Work out the finished part from the listing and answer in its coordinate system (mm). A direction names the side the tool comes from. Give positions to 0.01 mm unless a question says otherwise; leave off trailing zeros. Order: outer loops, then holes, each group sorted by start corner. A loop starts at its lowest first (then second) coordinate and runs counter-clockwise, first axis right, second up. Notation, with made-up numbers: (53.25, 76) -> (81.25, 76) arc R37 ccw to (81.25, 113) -> close; hole circle Ø1 at (-24.75, -14.5). An arc over 180 degrees is marked (long way). Use a Markdown table: item, result. Add a question column.
```python
from build123d import *

# Parameters (mm, degrees)
SKETCH1_W           = 14.8
SKETCH1_H           = 8.08
BOSS_EXTRUDE1_DEPTH = 6.94
FILLET1_SIZE        = 7
FILLET1_SIZE_2      = 3.4
SKETCH2_W           = 2.5
SKETCH2_H           = 5
BOSS_EXTRUDE2_DEPTH = 7.45
SKETCH3_W           = 4.44
SKETCH3_H           = 5
BOSS_EXTRUDE3_DEPTH = 3
CUT_EXTRUDE1_REACH  = 26.161
CUT_EXTRUDE2_REACH  = 26.161
CUT_EXTRUDE3_REACH  = 25.756
SKETCH6_W           = 1.27
SKETCH6_H           = 10.45
SKETCH7_W           = 6.5278
SKETCH7_H           = 5
SKETCH7_H_2         = 1.3
BOSS_EXTRUDE4_DEPTH = 2.55634
CUT_EXTRUDE4_REACH  = 24.207
SKETCH9_W           = 6.5278
SKETCH9_H           = 8.018408457
SKETCH9_W_2         = 4.3283
SKETCH9_H_2         = 5.8777
BOSS_EXTRUDE5_DEPTH = 16.3863


with BuildPart() as part:
    # Sketch1 → Boss-Extrude1 (new body)
    with BuildSketch(Plane(origin=(0, 0, 0), x_dir=(1, 0, 0), z_dir=(0, 1, 0))):
        with BuildLine():
            Line((0, -8.08), (14.8, -8.08))
            ThreePointArc((14.8, -8.08), (7.4, -15.48), (0, -8.08))
        make_face()
        with Locations((7.4, -4.04)):
            Rectangle(SKETCH1_W, SKETCH1_H)
        with BuildLine():
            ThreePointArc((0, 0), (7.4, 7.4), (14.8, 0))
            Line((14.8, 0), (0, 0))
        make_face()
    extrude(amount=BOSS_EXTRUDE1_DEPTH)

    # Fillet1
    # an asymmetric fillet: 7, 3.4 mm, written as the material it takes off along each edge
    with BuildSketch(Plane(origin=(7.4, 6.94, 0), x_dir=(-1, 0, 0), z_dir=(0, 0, 1))) as fillet1_piece_1:
        with BuildLine():
            Bezier((7.4 - FILLET1_SIZE, 0), (7.4, 0), (7.4, FILLET1_SIZE_2), weights=[1, 0.707106781, 1])
            Line((7.4, FILLET1_SIZE_2), (7.4, 0))
            Line((7.4, 0), (7.4 - FILLET1_SIZE, 0))
        make_face()
    revolve(axis=Axis((7.4, 6.94, 0), (0, -1, 0)), revolution_arc=180, mode=Mode.SUBTRACT)
    with BuildSketch(Plane(origin=(0, 6.94, 8.08), x_dir=(0, -1, 0), z_dir=(0, 0, -1)), Plane(origin=(14.8, 6.94, 0), x_dir=(0, -1, 0), z_dir=(0, 0, 1))) as fillet1_piece_2:
        with BuildLine():
            Bezier((FILLET1_SIZE_2, 0), (0, 0), (0, -FILLET1_SIZE), weights=[1, 0.707106781, 1])
            Line((0, -FILLET1_SIZE), (0, 0))
            Line((0, 0), (FILLET1_SIZE_2, 0))
        make_face()
    extrude(amount=8.08, mode=Mode.SUBTRACT)
    with BuildSketch(Plane(origin=(7.4, 6.94, 8.08), x_dir=(1, 0, 0), z_dir=(0, 0, -1))) as fillet1_piece_3:
        with BuildLine():
            Bezier((7.4, FILLET1_SIZE_2), (7.4, 0), (7.4 - FILLET1_SIZE, 0), weights=[1, 0.707106781, 1])
            Line((7.4 - FILLET1_SIZE, 0), (7.4, 0))
            Line((7.4, 0), (7.4, FILLET1_SIZE_2))
        make_face()
    revolve(axis=Axis((7.4, 6.94, 8.08), (0, -1, 0)), revolution_arc=180, mode=Mode.SUBTRACT)

    # Sketch2 → Boss-Extrude2 (add)
    with BuildSketch(Plane.XZ):
        with Locations((1.25, 4.04)):
            Rectangle(SKETCH2_W, SKETCH2_H)
        with Locations((13.55, 4.04)):
            Rectangle(SKETCH2_W, SKETCH2_H)
    extrude(amount=BOSS_EXTRUDE2_DEPTH)

    # Sketch3 → Boss-Extrude3 (add)
    with BuildSketch(Plane(origin=(0, -7.45, 0), x_dir=(-1, 0, 0), z_dir=(0, -1, 0))):
        with Locations((-0.28, -4.04)):
            Rectangle(SKETCH3_W, SKETCH3_H)
        with Locations((-14.52, -4.04)):
            Rectangle(SKETCH3_W, SKETCH3_H)
    extrude(amount=BOSS_EXTRUDE3_DEPTH)

    # Sketch4 → Cut-Extrude1 (cut, up to next)
    with BuildSketch(Plane(origin=(0, 0, 1.54), x_dir=(-1, 0, 0), z_dir=(0, 0, -1)), mode=Mode.PRIVATE) as cut_extrude1_sk1:
        Polygon((1.94, -7.45), (-0.28, -10.45), (1.94, -10.45), align=None)
    cut_extrude1_tool1 = extrude(cut_extrude1_sk1.sketch, amount=-CUT_EXTRUDE1_REACH, mode=Mode.PRIVATE) & part.part
    # Sketch4 → Cut-Extrude1 (cut, up to next)
    with BuildSketch(Plane(origin=(0, 0, 1.54), x_dir=(-1, 0, 0), z_dir=(0, 0, -1)), mode=Mode.PRIVATE) as cut_extrude1_sk2:
        Polygon((-16.74, -7.45), (-16.74, -10.45), (-14.52, -10.45), align=None)
    cut_extrude1_tool2 = extrude(cut_extrude1_sk2.sketch, amount=-CUT_EXTRUDE1_REACH, mode=Mode.PRIVATE) & part.part
    add(cut_extrude1_tool1.solids().sort_by_distance((-1.2, -9.45, 1.54))[0], mode=Mode.SUBTRACT)
    add(cut_extrude1_tool2.solids().sort_by_distance((16, -9.45, 1.54))[0], mode=Mode.SUBTRACT)

    # Sketch5 → Cut-Extrude2 (cut, up to next)
    with BuildSketch(Plane(origin=(0, 0, 1.54), x_dir=(-1, 0, 0), z_dir=(0, 0, -1)), mode=Mode.PRIVATE) as cut_extrude2_sk1:
        Polygon((-0.28, -10.45), (-0.87, -10.45), (1.35, -7.45), (1.94, -7.45), align=None)
    cut_extrude2_tool1 = extrude(cut_extrude2_sk1.sketch, amount=-CUT_EXTRUDE2_REACH, mode=Mode.PRIVATE) & part.part
    # Sketch5 → Cut-Extrude2 (cut, up to next)
    with BuildSketch(Plane(origin=(0, 0, 1.54), x_dir=(-1, 0, 0), z_dir=(0, 0, -1)), mode=Mode.PRIVATE) as cut_extrude2_sk2:
        Polygon((-14.52, -10.45), (-13.93, -10.45), (-16.15, -7.45), (-16.74, -7.45), align=None)
    cut_extrude2_tool2 = extrude(cut_extrude2_sk2.sketch, amount=-CUT_EXTRUDE2_REACH, mode=Mode.PRIVATE) & part.part
    add(cut_extrude2_tool1.solids().sort_by_distance((-0.535, -8.95, 1.54))[0], mode=Mode.SUBTRACT)
    add(cut_extrude2_tool2.solids().sort_by_distance((15.335, -8.95, 1.54))[0], mode=Mode.SUBTRACT)

    # Sketch6 → Cut-Extrude3 (cut, up to next)
    with BuildSketch(Plane(origin=(0, 0, 1.54), x_dir=(-1, 0, 0), z_dir=(0, 0, -1)), mode=Mode.PRIVATE) as cut_extrude3_sk1:
        with Locations((-1.865, -5.225)):
            Rectangle(SKETCH6_W, SKETCH6_H)
    cut_extrude3_tool1 = extrude(cut_extrude3_sk1.sketch, amount=-CUT_EXTRUDE3_REACH, mode=Mode.PRIVATE) & part.part
    # Sketch6 → Cut-Extrude3 (cut, up to next)
    with BuildSketch(Plane(origin=(0, 0, 1.54), x_dir=(-1, 0, 0), z_dir=(0, 0, -1)), mode=Mode.PRIVATE) as cut_extrude3_sk2:
        with Locations((-12.935, -5.225)):
            Rectangle(SKETCH6_W, SKETCH6_H)
    cut_extrude3_tool2 = extrude(cut_extrude3_sk2.sketch, amount=-CUT_EXTRUDE3_REACH, mode=Mode.PRIVATE) & part.part
    add(cut_extrude3_tool1.solids().sort_by_distance((1.865, -5.225, 1.54))[0], mode=Mode.SUBTRACT)
    add(cut_extrude3_tool2.solids().sort_by_distance((12.935, -5.225, 1.54))[0], mode=Mode.SUBTRACT)

    # Sketch7 → Boss-Extrude4 (add)
    with BuildSketch(Plane.XZ):
        with Locations((7.3989, 4.04)):
            Rectangle(SKETCH7_W, SKETCH7_H)
        with Locations((7.3989, 0.89)):
            Rectangle(SKETCH7_W, SKETCH7_H_2)
        with Locations((7.3989, 7.19)):
            Rectangle(SKETCH7_W, SKETCH7_H_2)
    extrude(amount=BOSS_EXTRUDE4_DEPTH)

    # Sketch8 → Cut-Extrude4 (cut, up to next)
    with BuildSketch(Plane(origin=(10.6628, 0, 0), x_dir=(0, 0, -1), z_dir=(1, 0, 0)), mode=Mode.PRIVATE) as cut_extrude4_sk1:
        Polygon((-0.24, -2.55634), (-7.84, 0), (-7.84, -2.55634), align=None)
    cut_extrude4_tool1 = extrude(cut_extrude4_sk1.sketch, amount=-CUT_EXTRUDE4_REACH, mode=Mode.PRIVATE) & part.part
    add(cut_extrude4_tool1.solids().sort_by_distance((10.6628, -1.704227, 5.306667))[0], mode=Mode.SUBTRACT)

    # Sketch9 → Boss-Extrude5 (add)
    with BuildSketch(Plane(origin=(0, -2.369037415, 0.796850672), x_dir=(1, 0, 0), z_dir=(0, -0.9478190142131836, 0.31880890247285915))):
        with Locations((7.3989, 3.421696842)):
            Rectangle(SKETCH9_W, SKETCH9_H)
        with Locations((7.3989, 3.421696843)):
            Rectangle(SKETCH9_W_2, SKETCH9_H_2, mode=Mode.SUBTRACT)
    extrude(amount=BOSS_EXTRUDE5_DEPTH)


solid = part.part
```
1) The part is cut by section C-C, the plane y = 2. Determine the outline of the cut face in (x, z).
2) Flat-ended cylindrical pins translate along their axes: pin 1 (2 mm diameter, centred on x = 12, y = 1, fed in from +Z); pin 2 (4 mm diameter, centred on y = -6, z = 3, fed in from -X); pin 3 (4 mm diameter, centred on y = -10, z = 7.5, fed in from -X); pin 4 (1 mm diameter, centred on x = 3.5, y = -11, fed in from +Z). Find the tip coordinate at first contact, or state that the pin passes through.
3) The part is cut by section A-A, the plane y = -5.5. Determine the outline of the cut face in (x, z) (3 decimals).
4) Which of the six approach directions +Z, -Z, +X, -X, +Y, -Y give full straight-line access (tool end or side, diameter ignored) to faces 4 (the flat face through (5.235, -9, 7)), 5 (the flat face through (1.23, -5, 4)), 6 (the flat face through (7.353, -7.657, 10.415)), 7 (the flat face through (15, -7.45, 4))?
5) Straight lines are drawn through the part: line 1 (X direction, y = -3.75, z = 4.25) (3 decimals); line 2 (X direction, y = -9.75, z = 4.25) (3 decimals); line 3 (X direction, y = -9.5, z = 8.25) (3 decimals). For each, find the intervals that lie inside material, in ascending order.
6) The part is cut by section B-B, the plane y = -14.75. Determine the outline of the cut face in (x, z) (3 decimals), then the cut area to 3 significant figures.
7) Determine the mould class of faces 1 (the cylindrical face through (7.56, 1.75, 15.48)), 2 (the flat face through (9.563, -9, 7)), 3 (the flat face through (10.663, -8, 6)) for opening direction Z: released by +Z, released by -Z, zero draft, split by the parting line, or undercut.
A:
| question | item | result |
|---|---|---|
| 1 | outline | (0, 0) arc R7.4 ccw to (14.8, 0) -> (14.8, 8.08) arc R7.4 ccw to (0, 8.08) -> close |
| 2 | pin 1 | z = 14.55 |
| 2 | pin 2 | x = -1.35 |
| 2 | pin 3 | x = -0.76 |
| 2 | pin 4 | through |
| 3 | outline | (0, 1.54) -> (1.23, 1.54) -> (1.23, 6.54) -> (0, 6.54) -> close; (4.135, 1.23) -> (10.663, 1.23) -> (10.663, 9.69) -> (4.135, 9.69) -> close; (13.57, 1.54) -> (14.8, 1.54) -> (14.8, 6.54) -> (13.57, 6.54) -> close; hole (5.235, 2.359) -> (9.563, 2.359) -> (9.563, 8.561) -> (5.235, 8.561) -> close |
| 4 | face 4 | none |
| 4 | face 5 | +Z, -Z, -Y |
| 4 | face 6 | +Z, +X, -X |
| 4 | face 7 | +Z, -Z, +X, +Y |
| 5 | line 1 | 0 to 1.23, 4.135 to 5.235, 9.563 to 10.663, 13.57 to 14.8 |
| 5 | line 2 | 0.352 to 1.23, 4.135 to 5.235, 9.563 to 10.663, 13.57 to 14.448 |
| 5 | line 3 | 4.135 to 5.235, 9.563 to 10.663 |
| 6 | outline | (4.135, 4.341) -> (10.663, 4.341) -> (10.663, 12.801) -> (4.135, 12.801) -> close; hole (5.235, 5.471) -> (9.563, 5.471) -> (9.563, 11.672) -> (5.235, 11.672) -> close |
| 6 | area | 28.4 mm^2 |
| 7 | face 1 | released by +Z |
| 7 | face 2 | undercut |
| 7 | face 3 | zero draft |
